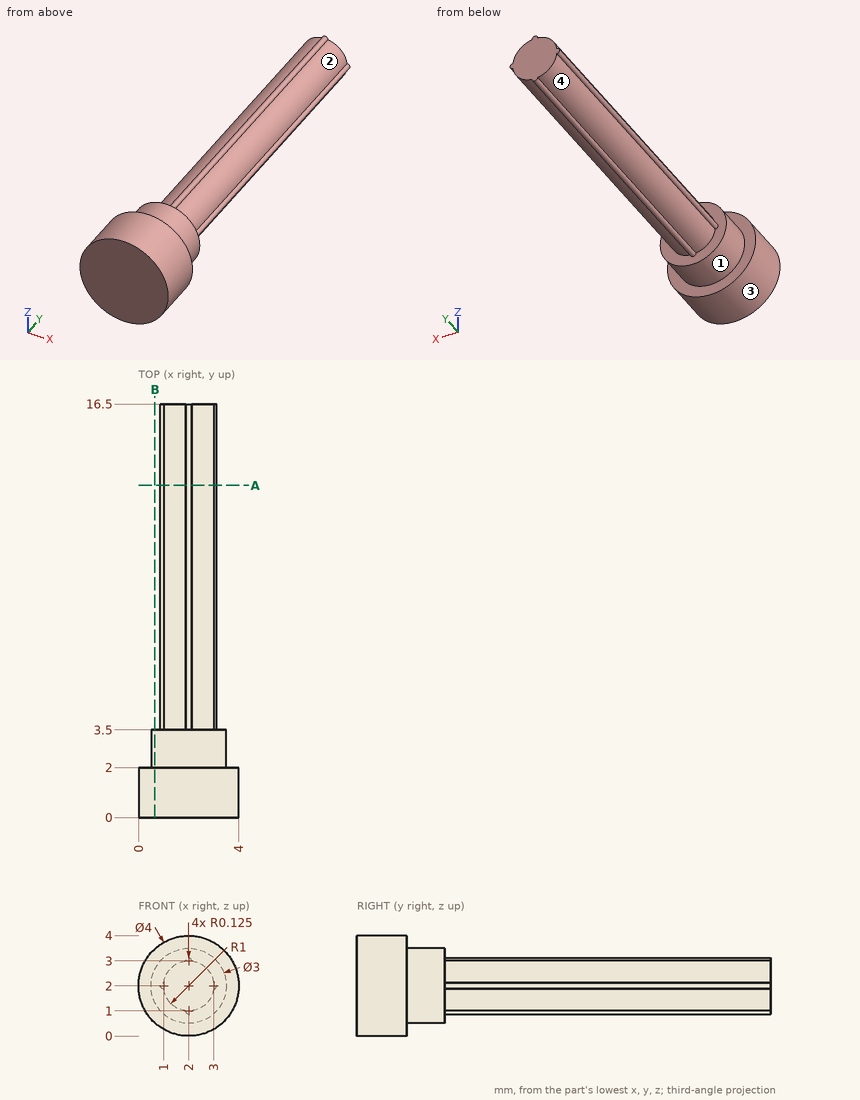
Drawing for the job (mm, zero at the part's lowest x, y, z). A direction names the side the tool comes from. Give positions to 0.01 mm unless a question says otherwise; leave off trailing zeros. Loops run counter-clockwise (first coordinate to the right, second up) from the corner with the lowest first, then second, coordinate; pieces in that order, holes last. Notation, with made-up numbers: M 80.25,77.25 L 110.25,77.25 A11 cw 110.25,89.25 Z; hole C 13,28 d6. An arc over 180 degrees is marked long. One line per question, with ' | ' between items. Start each with the question number.
1. Saw through at B-B on x = 0.65. Give the cut face in (y, z).
2. 3-axis set-ups, long thin cutter, end or side, ignore diameter. For the marked faces 1, 2, 3 and 4: which of +Z, -Z, +X, -X, +Y, -Y reach the whole face in a straight line?
3. Probe L1, parallel to Y at x = 3.1, z = 2.45; L2, parallel to Z at x = 2.3, y = 4.25; L3, parallel to Y at x = 2, z = 0.2. List the from-to ranges inside material, lowest first. Write a range as from..to.
4. Saw through at A-A on y = 13.25. Give the cut face in (x, z) (3 decimals), plus the area to 3 significant figures.
5. Flat gauge pin, fed straight in: pin 1 (2 mm diameter, centred on y = 7, z = 2, fed in from -X) (3 decimals). Where does the tip first touch, or does it go through?
Result sheet:
1) outline: M 0,0.52 L 2,0.52 L 2,1.35 L 3.5,1.35 L 3.5,2.65 L 2,2.65 L 2,3.48 L 0,3.48 Z
2) face 1: +Y | face 2: +Z, +X, +Y | face 3: +Y, -Y | face 4: -Z, -X, +Y
3) L1: y = 0..3.5 | L2: z = 1.05..2.95 | L3: y = 0..2
4) outline: M 1.008,1.875 A1 ccw 1.875,1.008 A0.125 ccw long 2.125,1.008 A1 ccw 2.992,1.875 A0.125 ccw long 2.992,2.125 A1 ccw 2.125,2.992 A0.125 ccw long 1.875,2.992 A1 ccw 1.008,2.125 A0.125 ccw long Z | area: 3.24 mm^2
5) pin 1: stops at x = 0.875
